Design review of the part built by this model. Coordinates are the model's own, in mm. A direction names the side the tool comes from. Give positions to 0.01 mm unless a question says otherwise; leave off trailing zeros. Write each loop counter-clockwise with the first axis right and the second up, starting at its lowest first coordinate (ties: lowest second). Pieces come first, ordered by that corner, then holes. Notation, with made-up numbers: (63.5, 72) -> (109.5, 72) arc R9 ccw to (109.5, 80) -> close; hole circle Ø6 at (35.5, 69). An arc over 180 degrees is marked (long way). Answer as a JSON object with one key per item and string values.
Autodesk Inventor part; units mm, degrees
ref_plane "YZ Plane" through (0, 0, 0) normal (1, 0, 0) x (0, 1, 0)
ref_plane "XZ Plane" through (0, 0, 0) normal (0, 1, 0) x (-1, 0, 0)
ref_plane "XY Plane" through (0, 0, 0) normal (0, 0, 1) x (1, 0, 0)
sketch "Szkic1" plane through (0, 0, 0) normal (0, 1, 0) x (-1, 0, 0)
  line L0 (-21, 18) -> (21, 18)
  line L1 (21, 18) -> (21, -18)
  line L2 (21, -18) -> (-21, -18)
  line L3 (-21, -18) -> (-21, 18)
  line L4 (-21, 18) -> (21, -18) construction
  line L5 (21, 18) -> (-21, -18) construction
  circle A0 centre (-15.25, -13) radius 2.75
  line L6 (0, 18) -> (0, -18)
  line L7 (-21, 0) -> (21, 0)
  circle A1 centre (-15.25, 13) radius 2.75
  line L8 (0, -18) -> (0, 18)
  circle A2 centre (15.25, -13) radius 2.75
  circle A3 centre (15.25, 13) radius 2.75
  line L9 (-21, -18) -> (20.4575, -18)
  line L10 (-21, -18) -> (21, -18)
  line L11 (21, -18) -> (21, -23)
  line L12 (21, -23) -> (-21, -23)
  line L13 (-21, -23) -> (-21, -18)
  circle A4 centre (0, -13.5) radius 4.5
  circle A5 centre (0, -13.5) radius 5.25
  line L14 (9, -18) -> (4.453, -10.7191)
  line L15 (-9, -18) -> (-4.453, -10.7191)
  point P0 (0, 0)
  point P1 (-21, -20.5)
  point P2 (0, -18)
  dimension "d11" = 10.5
  dimension "W12" = 42
  dimension "L12" = 36
  dimension "d2" = 5.5
  dimension "d3" = 5.75
  dimension "d4" = 5
  dimension "d6" = 5
  dimension "d7" = 42
  dimension "SrPopr" = 9
  dimension "d9" = 4.5
  dimension "d12" = 9
extrude "Wyciągnięcie proste1" add sketch "Szkic1" along normal blind 5
extrude "Wyciągnięcie proste2" add sketch "Szkic1" along normal blind 60 contours L2 A5 L11 L12 L13 | A5 L2 A4 L6 | L6 A4 L2 A5 | L15 A5 L2 | L14 L2 A5 | L2 A5
extrude "Wyciągnięcie proste3" cut sketch "Szkic1" along normal blind 50 contours A5 L2 A4 L6 | L6 A4 L2 A5 | L15 A5 L2 | L14 L2 A5
extrude "Wyciągnięcie proste4" add sketch "Szkic1" along normal blind 5 contours A5 L2 A4 L6 | L6 A4 L2 A5 | L15 A5 L2 | L14 L2 A5
sketch "Szkic3" plane through (-21, 5, -18) normal (0, 0, 1) x (1, 0, 0)
  line L0 (42, 0) -> (0, 0)
  line L1 (42, 0) -> (42, 55)
  line L2 (30, 55) -> (42, 55)
  line L3 (30, 45) -> (30, 55)
  line L4 (30, 45) -> (21, 45)
  line L5 (21, 45) -> (12, 45)
  line L6 (12, 45) -> (12, 55)
  line L7 (0, 55) -> (12, 55)
  line L8 (0, 0) -> (0, 55)
  line L9 (35, 42) -> (7, 42)
  line L10 (7, 42) -> (7, 0)
  line L11 (7, 0) -> (35, 0)
  line L12 (35, 0) -> (35, 42)
  line L13 (35, 42) -> (7, 0) construction
  line L14 (7, 42) -> (35, 0) construction
  line L15 (42, 0) -> (42, 55)
  line L16 (0, 0) -> (0, 55)
  line L17 (0, 0) -> (42, 0)
  line L18 (21, 0) -> (21, 42)
  line L19 (38, 0) -> (38, 45)
  line L20 (4, 45) -> (4, 0)
  line L21 (38, 45) -> (4, 45)
  line L22 (33.5, 0) -> (8.5, 0)
  line L23 (8.5, 0) -> (8.5, 10)
  line L24 (8.5, 10) -> (33.5, 10)
  line L25 (33.5, 10) -> (33.5, 0)
  line L26 (32, 42) -> (10, 42)
  line L27 (10, 42) -> (10, 32)
  line L28 (10, 32) -> (32, 32)
  line L29 (32, 32) -> (32, 42)
  line L30 (38, 20) -> (4, 20)
  point P0 (21, -5)
  point P1 (21, 21)
  point P2 (21, 0)
  point P3 (4, 0)
  point P4 (38, 0)
  point P5 (8.5, 0)
  point P6 (33.5, 0)
  point P7 (35, 20)
  point P8 (7, 20)
  dimension "d21" = 28
  dimension "d22" = 42
  dimension "GruboscAku" = 3
  dimension "d33" = 3
  dimension "d34" = 10
  dimension "d35" = 25
  dimension "d36" = 10
  dimension "d37" = 22
  dimension "d42" = 20
extrude "Wyciągnięcie proste5" add sketch "Szkic3" along normal blind 36 contours L30 L12 L9 L10 L20 L21 L5 L4 L19
extrude "Wyciągnięcie proste6" cut sketch "Szkic3" against normal blind 5 contours L0 L18 L24 L25 | L0 L23 L24 L18 | L29 L28 L18 L9 | L28 L27 L9 L18
extrude "Wyciągnięcie proste7" cut sketch "Szkic1" along normal blind 50 contours A4 L6 | L6 A4
extrude "Wyciągnięcie proste8" add sketch "Szkic1" along normal blind 5 contours A4 L6 | L6 A4
equation "\"d9\" = 0.5 * SrPopr"
equation "\"d33\" = GruboscAku"
properties part number "KatownikNowy"
(1) We need section C-C, the plane z = -1. State the section outline as (x, y) points.
Here are the results:
{"outline": "(-21, 0) -> (21, 0) -> (21, 5) -> (-21, 5) -> close; (-17, 25) -> (-14, 25) -> (-14, 47) -> (14, 47) -> (14, 25) -> (17, 25) -> (17, 50) -> (-17, 50) -> close"}
(2) We need section A-A, the plane y = 13. State the section outline as (x, z) points.
Here are the results:
{"outline": "(-21, -23) -> (-12.5, -23) -> (-12.5, -18) -> (-21, -18) -> close; (12.5, -23) -> (21, -23) -> (21, -18) -> (12.5, -18) -> close"}
(3) Clearance check with flat-ended pins moving along their axes: pin 1 (7.5 mm diameter, centred on y = 43.5, z = 4, fed in from -X); pin 2 (2 mm diameter, centred on x = 2, z = -3, fed in from -Y); pin 3 (1.5 mm diameter, centred on x = 10.5, z = -17, fed in from +Y); pin 4 (11 mm diameter, centred on y = 31, z = 2, fed in from +X). State where each tip first meets the part, or that it passes through.
Here are the results:
{"pin 1": "stops at x = -17", "pin 2": "stops at y = 0", "pin 3": "stops at y = 50", "pin 4": "stops at x = 17"}
(4) We need section B-B, the plane x = 0. State the section outline as (y, z) points, then the cut area to 4 significant figures.
Here are the results:
{"outline": "(0, -23) -> (5, -23) -> (5, 18) -> (0, 18) -> close; (15, -23) -> (37, -23) -> (37, -18) -> (15, -18) -> close; (47, -23) -> (60, -23) -> (60, -18) -> (47, -18) -> close; (47, -9) -> (60, -9) -> (60, -8.25) -> (50, -8.25) -> (50, 18) -> (47, 18) -> close", "area": "468.5 mm²"}
(5) The part is to be moulded in two halves that separate along X. For faces 4 (the flat face through (11, 42, -20)), 5 (the flat face through (-21, 19, -19)), 6 (the flat face through (17, 37, 0)), 7 (the flat face through (0, 32, -18)), say which applies: +X half, -X half, draft (parallel to the pull), parting line (faces both ways), or undercut.
Here are the results:
{"face 4": "undercut", "face 5": "-X half", "face 6": "+X half", "face 7": "undercut"}
(6) For faces 1 (the flat face through (-17, 38, 0)), 2 (the flat face through (0, 37, -20)), 3 (the flat face through (0, 50, 0)), list the 3-axis set-ups (+Z, -Z, +X, -X, +Y, -Y) from which the entire face can be reached by the end or side of a thin tool; tool diameter is ignored.
Here are the results:
{"face 1": "+Z, -X, +Y", "face 2": "+Z, -Z", "face 3": "+Z, +Y"}
(7) We need section D-D, the plane z = 13. State the section outline as (x, y) points.
Here are the results:
{"outline": "(-21, 0) -> (-18, 0) -> (-18, 5) -> (-21, 5) -> close; (-17, 25) -> (-14, 25) -> (-14, 47) -> (14, 47) -> (14, 25) -> (17, 25) -> (17, 50) -> (-17, 50) -> close; (-12.5, 0) -> (12.5, 0) -> (12.5, 5) -> (-12.5, 5) -> close; (18, 0) -> (21, 0) -> (21, 5) -> (18, 5) -> close"}
(8) For line 1 along Z through (x, y) = (15, 1); line 2 along Y through (x, z) = (16, 6); line 3 along Y through (x, z) = (-11, -3), list the stretches that pass through material, from the lowest coordinate up.
Here are the results:
{"line 1": "z = -23 to -15.74, -10.26 to 10.26, 15.74 to 18", "line 2": "y = 0 to 5, 25 to 50", "line 3": "y = 0 to 5, 47 to 50"}
